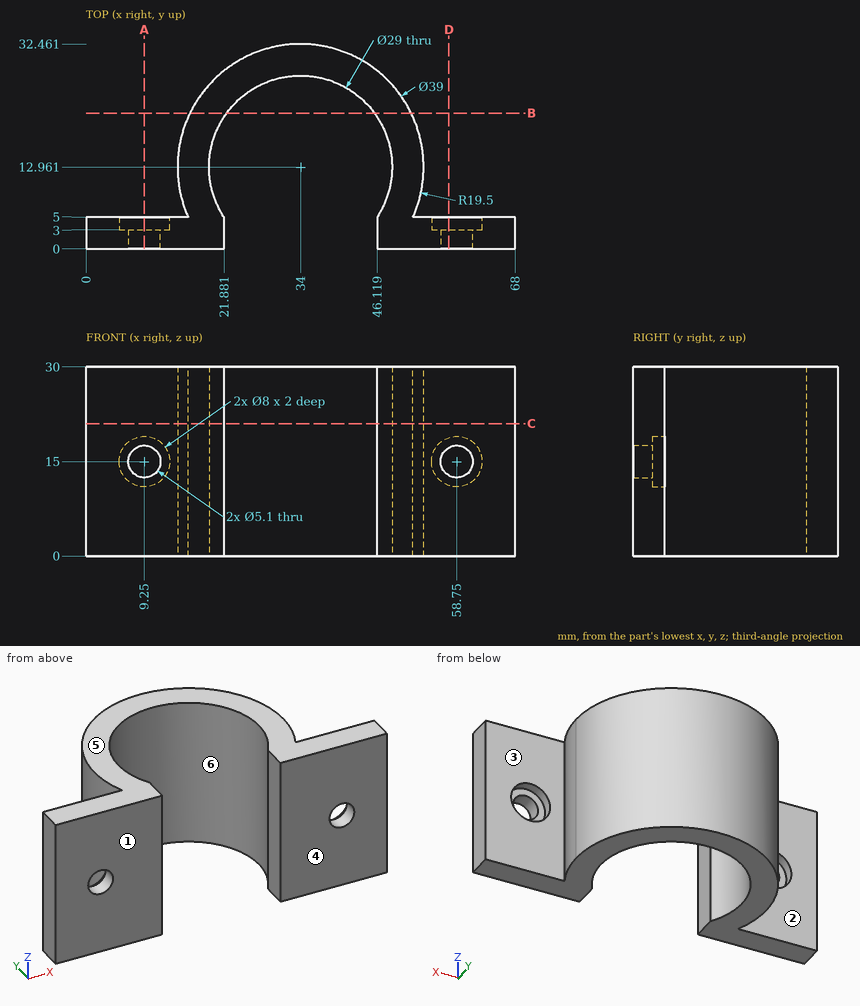
Design review of the part shown in the three views and the two pictorial views. Dimensions are in mm from the part's minimum x, y and z. A direction names the side the tool comes from. Round coordinates to 2 decimals unless told otherwise and drop trailing zeros. Write each loop counter-clockwise with the first axis right and the second up, starting at its lowest first coordinate (ties: lowest second). Pieces come first, ordered by that corner, then holes. Notation, with made-up numbers: (23, 64) -> (82, 64) arc R26 ccw to (82, 88) -> close; hole circle Ø11 at (-12.75, 86). An arc over 180 degrees is marked (long way). Answer as a JSON object with one key per item and string values.
1. Machinability: for the marked faces 1, 2 and 3, which of the approach directions +Z, -Z, +X, -X, +Y, -Y give a long, thin tool a straight path to every point of the face, cutting with its end or side? Answer none if there is none.
Results found:
{"face 1": "+Z, -Z, +X, -X, -Y", "face 2": "+Z, -Z, -X", "face 3": "+Z, -Z, +X"}
2. Clearance check with flat-ended pins moving along their axes: pin 1 (9 mm diameter, centred on x = 7.5, z = 15, fed in from +Y); pin 2 (8 mm diameter, centred on x = 15.5, y = 14, fed in from -Z); pin 3 (18 mm diameter, centred on x = 12, z = 14, fed in from +Y) (1 decimal); pin 4 (6.5 mm diameter, centred on x = 9.25, z = 15, fed in from +Y). State where each tip first meets the part, or that it passes through.
Results found:
{"pin 1": "stops at y = 5", "pin 2": "stops at z = 0", "pin 3": "stops at y = 27.5", "pin 4": "stops at y = 3"}
3. We need section B-B on y = 21.5. State the section outline as (x, z) points.
Results found:
{"outline": "(16.47, 0) -> (22.28, 0) -> (22.28, 30) -> (16.47, 30) -> close; (45.72, 0) -> (51.53, 0) -> (51.53, 30) -> (45.72, 30) -> close"}
4. We need section D-D on x = 57.5. State the section outline as (y, z) points.
Results found:
{"outline": "(0, 0) -> (5, 0) -> (5, 11.2) -> (3, 11.2) -> (3, 12.78) -> (0, 12.78) -> close; (0, 17.22) -> (3, 17.22) -> (3, 18.8) -> (5, 18.8) -> (5, 30) -> (0, 30) -> close"}
5. The part is to be moulded in two halves that separate along Y. For the marked faces 4, 5 and 6, say which applies: pulls with the +Y half, pulls with the -Y half, needs draft (parallel to the pull), parting line crosses it, or undercut.
Results found:
{"face 4": "pulls with the -Y half", "face 5": "needs draft", "face 6": "undercut"}
6. We need section A-A on x = 9.25. State the section outline as (y, z) points, and give its area (3 significant figures).
Results found:
{"outline": "(0, 0) -> (5, 0) -> (5, 11) -> (3, 11) -> (3, 12.45) -> (0, 12.45) -> close; (0, 17.55) -> (3, 17.55) -> (3, 19) -> (5, 19) -> (5, 30) -> (0, 30) -> close", "area": "119 mm^2"}
7. To check wall thickness, follow line 1 along Z through (x, y) = (58.75, 3.85); line 2 along X through (y, z) = (3, 24); line 3 along Z through (x, y) = (9.25, 1.55). State the ranges of each line that lie inside material, in increasing order.
Results found:
{"line 1": "z = 0 to 11, 19 to 30", "line 2": "x = 0 to 21.88, 46.12 to 68", "line 3": "z = 0 to 12.45, 17.55 to 30"}
8. We need section C-C on z = 21. State the section outline as (x, y) points, and give its area (3 significant figures).
Results found:
{"outline": "(0, 0) -> (21.88, 0) -> (21.88, 5) arc R14.5 cw (long way) to (46.12, 5) -> (46.12, 0) -> (68, 0) -> (68, 5) -> (51.8, 5) arc R19.5 ccw (long way) to (16.2, 5) -> (0, 5) -> close", "area": "569 mm^2"}
